from build123d import *

# Parameters (mm, degrees)
F0_W     = 22
F0_H     = 36
F0_W_2   = 12
F0_H_2   = 26
F1_DEPTH = 24.5
F2_DEPTH = 2
F3_R     = 1
F4_DEPTH = 36.001


with BuildPart() as f1:
    # F0 (on Top) → F1 (new body)
    with BuildSketch(Plane.XY):
        with Locations((6, -13)):
            Rectangle(F0_W, F0_H)
        with Locations((6, -13)):
            Rectangle(F0_W_2, F0_H_2, mode=Mode.SUBTRACT)
    extrude(amount=F1_DEPTH)

    # F0 (on Top) → F2 (join)
    with BuildSketch(Plane.XY):
        with Locations((6, -13)):
            Rectangle(F0_W_2, F0_H_2)
    extrude(amount=F2_DEPTH)

    # F3 (on face) → F4 (cut, through all)
    with BuildSketch(Plane.XZ.offset(31)):
        with Locations((5.945511, 5.631423)):
            Circle(F3_R)
    extrude(amount=-F4_DEPTH, mode=Mode.SUBTRACT)


solid = f1.part
Geometry check sheet. Reference: the model listing, model coordinates, mm. A direction names the side the tool comes from. Round coordinates to 2 decimals unless told otherwise and drop trailing zeros. Write each loop counter-clockwise with the first axis right and the second up, starting at its lowest first coordinate (ties: lowest second). Pieces come first, ordered by that corner, then holes.
Item 1: Section check B-B (z = 9.25). Record the boundary of the cut face in (x, y), plus the area to 3 significant figures.
Determined:
outline: (-5, -31) - (17, -31) - (17, 5) - (-5, 5) - close; hole (0, -26) - (12, -26) - (12, 0) - (0, 0) - close
area: 480 mm2
Item 2: Go/stop test with flat-tipped pins: pin 1 Ø1.8 at (x, z) = (5.95, 5.63) entering from -Y; pin 2 Ø1.5 at (x, y) = (4.5, -14.5) entering from +Z. Record where each tip stops, or that it passes through.
Determined:
pin 1: passes through
pin 2: stops at z = 2
Item 3: Section check C-C (x = 8.5). Record the boundary of the cut face in (y, z), plus the area to 3 significant figures.
Determined:
outline: (-31, 0) - (5, 0) - (5, 24.5) - (0, 24.5) - (0, 2) - (-26, 2) - (-26, 24.5) - (-31, 24.5) - close
area: 297 mm2
Item 4: Section check D-D (x = 6.25). Record the boundary of the cut face in (y, z), plus the area to 3 significant figures.
Determined:
outline: (-31, 0) - (5, 0) - (5, 4.68) - (0, 4.68) - (0, 2) - (-26, 2) - (-26, 4.68) - (-31, 4.68) - close; (-31, 6.58) - (-26, 6.58) - (-26, 24.5) - (-31, 24.5) - close; (0, 6.58) - (5, 6.58) - (5, 24.5) - (0, 24.5) - close
area: 278 mm2
Item 5: Section check A-A (y = -22.5). Record the boundary of the cut face in (x, z), plus the area to 3 significant figures.
Determined:
outline: (-5, 0) - (17, 0) - (17, 24.5) - (12, 24.5) - (12, 2) - (0, 2) - (0, 24.5) - (-5, 24.5) - close
area: 269 mm2
Item 6: Mould release check, pull along Y, two halves, no side actions. Record for faces 3 (the face through (0, -13, 13)), 4 (the face through (13, -13, 24.5)), 5 (the face through (6, -31, 12)), 6 (the face through (12, -13, 13)): +Y half, -Y half, draft (parallel to the pull), parting line (faces both ways), or undercut.
Determined:
face 3: undercut
face 4: draft
face 5: -Y half
face 6: undercut
Item 7: Material ranges on line 1 along X through (y, z) = (-13.5, 12.75); line 2 along Y through (x, z) = (10.75, 11.5); line 3 along Z through (x, y) = (2.75, -1), recorded low to high.
Determined:
line 1: x = -5 to 0, 12 to 17
line 2: y = -31 to -26, 0 to 5
line 3: z = 0 to 2
Item 8: Access from +Z, -Z, +X, -X, +Y, -Y to the whole of each face (thin tool, end or side, straight path). Record for faces 1 (the face through (6, -13, 2)), 2 (the face through (17, -13, 12)).
Determined:
face 1: +Z
face 2: +Z, -Z, +X, +Y, -Y
